Verification items for the finished model (mm, model axes). A direction names the side the tool comes from. Coordinates: 2 decimals unless noted, no trailing zeros. Loops run counter-clockwise (first coordinate to the right, second up) from the corner with the lowest first, then second, coordinate; pieces in that order, holes last. Notation, with made-up numbers: M -19.75,33.25 L 30.25,33.25 A14 ccw 30.25,51.25 Z; hole C 89.5,6 d4. An arc over 180 degrees is marked long. Write item = value, one per line. Start each with the question number.
```python
from build123d import *

# Parameters (mm, degrees)
SKETCH_1_W          = 110
SKETCH_1_H          = 50
EXTRUDE_1_DEPTH     = 3
EXTRUDE_2_DEPTH     = 45
SKETCH_6_R          = 2
EXTRUDE_986_DEPTH   = 10
CUT_EXTRUDE_1_DEPTH = 42
SKETCH_8_W          = 84
SKETCH_8_H          = 3
EXTRUDE_3_DEPTH     = 15
FILLET_1_R          = 1.5


with BuildPart() as part:
    # 草图1 → 凸台-拉伸1 (new body)
    with BuildSketch(Plane(origin=(0, 0, 0), x_dir=(1, 0, 0), z_dir=(0, 1, 0))):
        Rectangle(SKETCH_1_W, SKETCH_1_H)
    extrude(amount=EXTRUDE_1_DEPTH)

    # 草图2 → 凸台-拉伸2 (add, symmetric)
    with BuildSketch(Plane(origin=(0, 0, 0), x_dir=(0, 0, -1), z_dir=(1, 0, 0))):
        with BuildLine():
            Line((-17.5, 0), (-17.5, -22))
            ThreePointArc((-17.5, -22), (4.029354416, -17.410336571), (17.5, 0))
            Line((17.5, 0), (-17.5, 0))
        make_face()
    extrude(amount=EXTRUDE_2_DEPTH, both=True)

    # 草图6 → Extrude 986 (add)
    with BuildSketch(Plane.XZ):
        with Locations(Location((-51, 20, 0), (0, 0, 270))):
            Circle(SKETCH_6_R)
        with Locations(Location((-51, -20, 0), (0, 0, 90))):
            Circle(SKETCH_6_R)
        with Locations(Location((51, 20, 0), (0, 0, 90))):
            Circle(SKETCH_6_R)
        with Locations(Location((51, -20, 0), (0, 0, 270))):
            Circle(SKETCH_6_R)
    extrude(amount=EXTRUDE_986_DEPTH)

    # 草图7 → 切除-拉伸1 (cut, symmetric)
    with BuildSketch(Plane(origin=(0, 0, 0), x_dir=(0, 0, -1), z_dir=(1, 0, 0))):
        with BuildLine():
            Line((-14.5, 3), (-14.5, -19.279154905))
            ThreePointArc((-14.5, -19.279154905), (4.394615248, -13.521903359), (15.219546663, 3))
            Line((15.219546663, 3), (-14.5, 3))
        make_face()
    extrude(amount=CUT_EXTRUDE_1_DEPTH, both=True, mode=Mode.SUBTRACT)

    # 草图8 → 凸台-拉伸3 (add)
    with BuildSketch(Plane(origin=(0, 0, 14.5), x_dir=(-1, 0, 0), z_dir=(0, 0, -1))):
        with Locations((0, 1.5)):
            Rectangle(SKETCH_8_W, SKETCH_8_H)
    extrude(amount=EXTRUDE_3_DEPTH)

    # 圆角1
    fillet_1_edges = [part.edges().sort_by_distance(p)[0] for p in [
        (0, 0, -0.5),
        (0, 3, -0.5),
    ]]
    fillet(fillet_1_edges, radius=FILLET_1_R - 0.0001)  # a hair under: the kernel refuses the full size


solid = part.part
```
Q1. Sectioned sample at A-A on y = -6. Record the cut outline in (x, z), plus the area to 3 significant figures.
Q2. Set-up check for faces 4 (the face through (1, 0, 8)), 5 (the face through (-45, -9, 4)), 6 (the face through (45, -9, 4)): record each of +Z, -Z, +X, -X, +Y, -Y from which the full face is reachable in a straight line by a thin tool's end or side.
Q3. Sectioned sample at C-C on z = -20. Record the cut outline in (x, y).
Q4. Scan lines: L1, parallel to X at y = -13, z = 3; L2, parallel to Y at x = -15, z = 14; L3, parallel to Z at x = 39, y = -5.75. Record each from-to range of solid material in increasing order. Write a range as [from, to].
Q5. Mould release check, pull along Y, two halves, no side actions. Record for faces 1 (the face through (51, -10, -20)), 2 (the face through (-53, -5, 20)), 3 (the face through (42, -8, 3)): +Y half, -Y half, draft (parallel to the pull), parting line (faces both ways), or undercut.
Q6. Sectioned sample at D-D on y = -11. Record the cut outline in (x, z).
Q7. Gauge pin test, flat ends, axial feed: pin 1 (5 mm diameter, centred on x = -41.5, y = -12, fed in from +Z); pin 2 (2 mm diameter, centred on x = 51.5, z = 20, fed in from -Y); pin 3 (3 mm diameter, centred on x = -6, y = -1, fed in from +Z); pin 4 (11 mm diameter, centred on y = -6.5, z = -6.5, fed in from -X). Record the tip position at first contact, or that the pin passes through.
Solutions:
q1.outline = C -51,-20 d4; C -51,20 d4; M -45,-14.89 L 45,-14.89 L 45,17.5 L -45,17.5 Z; C 51,-20 d4; C 51,20 d4; hole M -42,-11.39 L 42,-11.39 L 42,14.5 L -42,14.5 Z
q1.area = 791 mm²
q2.face_4 = none
q2.face_5 = +Z, -Z, -X, -Y
q2.face_6 = +Z, -Z, +X, -Y
q3.outline = M -55,0 L -53,0 L -53,-10 L -49,-10 L -49,0 L 49,0 L 49,-10 L 53,-10 L 53,0 L 55,0 L 55,3 L -55,3 Z
q4.L1 = [-45, -42], [42, 45]
q4.L2 = [-22.3, -19.3], [0, 3]
q4.L3 = [-15.03, -11.55], [14.5, 17.5]
q5.face_1 = -Y half
q5.face_2 = draft
q5.face_3 = undercut
q6.outline = M -45,-11.42 L 45,-11.42 L 45,17.5 L -45,17.5 Z; hole M -42,-7.33 L 42,-7.33 L 42,14.5 L -42,14.5 Z
q7.pin_1 = 17.5
q7.pin_2 = -10
q7.pin_3 = 25
q7.pin_4 = -45
